Geometry check sheet. Reference: the model listing, model coordinates, mm. A direction names the side the tool comes from. Give positions to 0.01 mm unless a question says otherwise; leave off trailing zeros. Write each loop counter-clockwise with the first axis right and the second up, starting at its lowest first coordinate (ties: lowest second). Pieces come first, ordered by that corner, then holes. Notation, with made-up numbers: (60.25, 78.25) -> (84.25, 78.25) arc R8 cw to (84.25, 93.25) -> close; hole circle Ø5 at (-20.5, -32). An arc over 180 degrees is marked (long way). Write item = value, one per line. Start each with the question number.
1. Depth check by flat-ended pin: P1, Ø3, axis at x = 35.5, z = 2.5, coming from the +Y side; P2, Ø1.5, axis at y = 0.5, z = -2.5, coming from the -X side; P3, Ø6, axis at x = 14.5, z = 0.5, coming from the +Y side; P4, Ø8, axis at x = 34.5, z = -0.5, coming from the -Y side. Enter the tip coordinate at first touch or a pass-through.
2. Cross-section at B-B, the plane y = 0. Record the cut outline in (x, z), plus the area to 3 significant figures.
3. Cross-section at C-C, the plane x = 4.5. Record the cut outline in (y, z).
4. Set-up check for faces 1 (the flat face through (30, -9, 0)), 2 (the flat face through (0, 0, 0)), 3 (the flat face through (30, 9, 0)), 4 (the flat face through (8, -9, -5)): record each of +Z, -Z, +X, -X, +Y, -Y from which the full face is reachable in a straight line by a thin tool's end or side.
5. Cross-section at D-D, the plane x = 9. Record the cut outline in (y, z).
6. Cross-section at A-A, the plane z = 0. Record the cut outline in (x, y), plus the area to 3 significant figures.
7. Thickness scan on line 1 along Z through (x, y) = (14, 8.5); line 2 along X through (y, z) = (-10.5, 2.5); line 3 along Y through (x, z) = (36, 1.5). Record the ranges inside material, lowest first.
```python
from build123d import *

# Parameters (mm, degrees)
CHAMFER1_SIZE      = 1
CUT_EXTRUDE1_DEPTH = 10


with BuildPart() as part:
    # Sketch1 → Revolve1 (revolve)
    with BuildSketch(Plane.XY, mode=Mode.PRIVATE) as revolve1_sk:
        Polygon((0, 0), (0, 13), (8, 13), (8, 10), (40, 10), (40, 0), align=None)
    revolve(revolve1_sk.sketch.rotate(Axis((0, 0, 0), (1, 0, 0)), 90), axis=Axis((0, 0, 0), (1, 0, 0)))

    # Chamfer1
    chamfer1_edges = [part.edges().sort_by_distance(p)[0] for p in [
        (40, 0, -10),
        (8, 0, -13),
        (0, 0, -13),
    ]]
    chamfer(chamfer1_edges, length=CHAMFER1_SIZE)

    # Sketch2 → Cut-Extrude1 (cut)
    with BuildSketch(Plane(origin=(40, 0, 0), x_dir=(0, 0, -1), z_dir=(1, 0, 0))):
        with BuildLine():
            ThreePointArc((5.267826876, 8.5), (0, 10), (-5.267826876, 8.5))
            Line((-5.267826876, 8.5), (-2.958039892, 8.5))
            ThreePointArc((-2.958039892, 8.5), (0, 9), (2.958039892, 8.5))
            Line((2.958039892, 8.5), (5.267826876, 8.5))
        make_face()
        with BuildLine():
            ThreePointArc((2.958039892, 8.5), (0, 9), (-2.958039892, 8.5))
            Line((-2.958039892, 8.5), (2.958039892, 8.5))
        make_face()
        with BuildLine():
            Line((-2.958039892, -8.5), (-5.267826876, -8.5))
            ThreePointArc((-5.267826876, -8.5), (0, -10), (5.267826876, -8.5))
            Line((5.267826876, -8.5), (2.958039892, -8.5))
            ThreePointArc((2.958039892, -8.5), (0, -9), (-2.958039892, -8.5))
        make_face()
        with BuildLine():
            Line((2.958039892, -8.5), (-2.958039892, -8.5))
            ThreePointArc((-2.958039892, -8.5), (0, -9), (2.958039892, -8.5))
        make_face()
    extrude(amount=-CUT_EXTRUDE1_DEPTH, mode=Mode.SUBTRACT)


solid = part.part
```
Answers:
q1.P1 = 8.5
q1.P2 = 0
q1.P3 = 10
q1.P4 = -8.5
q2.outline = (0, -12) -> (1, -13) -> (7, -13) -> (8, -12) -> (8, -10) -> (39, -10) -> (40, -9) -> (40, 9) -> (39, 10) -> (8, 10) -> (8, 12) -> (7, 13) -> (1, 13) -> (0, 12) -> close
q2.area = 845 mm^2
q3.outline = circle Ø26 at (0, 0)
q4.face_1 = +Z, -Z, +X, -Y
q4.face_2 = +Z, -Z, -X, +Y, -Y
q4.face_3 = +Z, -Z, +X, +Y
q4.face_4 = +X
q5.outline = circle Ø20 at (0, 0)
q6.outline = (0, -12) -> (1, -13) -> (7, -13) -> (8, -12) -> (8, -10) -> (30, -10) -> (30, -8.5) -> (40, -8.5) -> (40, 8.5) -> (30, 8.5) -> (30, 10) -> (8, 10) -> (8, 12) -> (7, 13) -> (1, 13) -> (0, 12) -> close
q6.area = 816 mm^2
q7.line_1 = -5.27 to 5.27
q7.line_2 = 0 to 8
q7.line_3 = -8.5 to 8.5
